from build123d import *

# Parameters (mm, degrees)
SKETCH1_W                                   = 65
SKETCH1_H                                   = 40
BOSS_EXTRUDE1_DEPTH                         = 30
SKETCH3_R                                   = 10
CUT_EXTRUDE2_DEPTH                          = 35
CBORE_FOR_M4_CHEESE_HEAD_SCREW1_D           = 4.5
CBORE_FOR_M4_CHEESE_HEAD_SCREW1_CBORE_D     = 8
CBORE_FOR_M4_CHEESE_HEAD_SCREW1_CBORE_DEPTH = 2.6
SKETCH10_R                                  = 2.25
CUT_EXTRUDE8_DEPTH                          = 4
CUT_EXTRUDE9_DEPTH                          = 15
CUT_EXTRUDE10_DEPTH                         = 83.006097414
FILLET9_R                                   = 8
SKETCH12_R                                  = 2.25
CUT_EXTRUDE11_DEPTH                         = 8
SKETCH12_3_R                                = 2.25
CUT_EXTRUDE12_DEPTH                         = 79.010807554
FILLET10_R                                  = 3


with BuildPart() as part:
    # Sketch1 → Boss-Extrude1 (new body)
    with BuildSketch(Plane(origin=(0, 0, 0), x_dir=(1, 0, 0), z_dir=(0, 1, 0))):
        with Locations((32.5, 20)):
            Rectangle(SKETCH1_W, SKETCH1_H)
    extrude(amount=BOSS_EXTRUDE1_DEPTH)

    # Sketch3 → Cut-Extrude2 (cut)
    with BuildSketch(Plane(origin=(65, 0, 0), x_dir=(0, 0, -1), z_dir=(1, 0, 0))):
        with Locations((20, 15)):
            Circle(SKETCH3_R)
    extrude(amount=-CUT_EXTRUDE2_DEPTH, mode=Mode.SUBTRACT)

    # CBORE for M4 Cheese Head Screw1 (through all)
    with Locations(Plane(origin=(0, 30, 0), x_dir=(1, 0, 0), z_dir=(0, 1, 0))):
        with Locations((53, 20)):
            CounterBoreHole(CBORE_FOR_M4_CHEESE_HEAD_SCREW1_D / 2, CBORE_FOR_M4_CHEESE_HEAD_SCREW1_CBORE_D / 2, CBORE_FOR_M4_CHEESE_HEAD_SCREW1_CBORE_DEPTH)

    # Sketch10 → Cut-Extrude8 (cut)
    with BuildSketch(Plane.XZ):
        Polygon((53, -15.669872981), (49.25, -17.834936491), (49.25, -22.165063509), (53, -24.330127019), (56.75, -22.165063509), (56.75, -17.834936491), align=None)
        with Locations(Location((53, -20, 0), (0, 0, 90))):
            Circle(SKETCH10_R, mode=Mode.SUBTRACT)
    extrude(amount=-CUT_EXTRUDE8_DEPTH, mode=Mode.SUBTRACT)

    # Sketch2 → Cut-Extrude9 (cut)
    with BuildSketch(Plane(origin=(0, 30, 0), x_dir=(1, 0, 0), z_dir=(0, 1, 0))):
        with BuildLine():
            Line((17.014944168, 22.55), (12.985055832, 22.55))
            ThreePointArc((12.985055832, 22.55), (13.583325822, 17.075015509), (18.25, 20))
            ThreePointArc((18.25, 20), (17.924984491, 21.416674178), (17.014944168, 22.55))
        make_face()
    extrude(amount=-CUT_EXTRUDE9_DEPTH, mode=Mode.SUBTRACT)

    # Sketch2<7> → Cut-Extrude10 (cut, through all)
    with BuildSketch(Plane(origin=(0, 30, 0), x_dir=(1, 0, 0), z_dir=(0, 1, 0))):
        with BuildLine():
            Line((65, 40), (0, 40))
            Line((0, 40), (0, 19.999999921))
            ThreePointArc((0, 19.999999921), (4.393398254, 30.60660169), (15, 35))
            add(Edge.make_bspline(
                [(15, 35), (30.758528256, 35), (45.015961289, 29.236867717), (65, 40)],
                knots=[0, 0, 0, 0, 1, 1, 1, 1], degree=3))
        make_face()
        with BuildLine():
            ThreePointArc((15, 5), (4.39339831, 9.393398254), (0, 19.999999921))
            Line((0, 19.999999921), (0, 0))
            Line((0, 0), (65, 0))
            add(Edge.make_bspline(
                [(15, 5), (30.758528256, 5), (45.015961289, 10.763132283), (65, 0)],
                knots=[0, 0, 0, 0, 1, 1, 1, 1], degree=3))
        make_face()
    extrude(amount=-CUT_EXTRUDE10_DEPTH, mode=Mode.SUBTRACT)

    # Fillet9
    # the kernel refuses this fillet: 8 mm, written as the material it takes off along each edge
    with BuildSketch(Plane(origin=(65, 0, -40), x_dir=(0, 0, 1), z_dir=(0, 1, 0))) as fillet9_piece_1:
        with BuildLine():
            CenterArc((12.0050638, -8), FILLET9_R, 90, 106.898701243)
            Line((4.350502414, -10.325444039), (4.197411186, -10.37195292))
            ThreePointArc((4.197411186, -10.37195292), (2.285588644, -5.115947892), (-0.140868031, -0.075869611))
            Line((-0.140868031, -0.075869611), (0, 0.16))
            Line((0, 0.16), (12.0050638, 0.16))
            Line((12.0050638, 0.16), (12.0050638, 0))
        make_face()
    extrude(amount=30, mode=Mode.SUBTRACT)
    with BuildSketch(Plane(origin=(65, 0, 0), x_dir=(0, 0, -1), z_dir=(0, 1, 0))) as fillet9_piece_2:
        with BuildLine():
            CenterArc((12.0050638, 8), FILLET9_R, 163.101298757, 106.898701243)
            Line((4.350502414, 10.325444039), (4.197411186, 10.37195292))
            ThreePointArc((4.197411186, 10.37195292), (2.285588644, 5.115947892), (-0.140868031, 0.075869611))
            Line((-0.140868031, 0.075869611), (0, -0.16))
            Line((0, -0.16), (12.0050638, -0.16))
            Line((12.0050638, -0.16), (12.0050638, 0))
        make_face()
    extrude(amount=30, mode=Mode.SUBTRACT)

    # Sketch12 → Cut-Extrude11 (cut)
    # profile 1 of 2: a face of its own
    with BuildSketch(Plane.XY.offset(-35)):
        Polygon((15, 17.727608008), (18.7, 19.863804004), (18.7, 24.136195996), (15, 26.272391992), (11.3, 24.136195996), (11.3, 19.863804004), align=None)
        with Locations((15, 22)):
            Circle(SKETCH12_R, mode=Mode.SUBTRACT)
    # profile 2 of 2: a face of its own
    with BuildSketch(Plane.XY.offset(-35)):
        with Locations((15, 22)):
            Circle(SKETCH12_R)
    extrude(amount=CUT_EXTRUDE11_DEPTH, mode=Mode.SUBTRACT)

    # Sketch12<3> → Cut-Extrude12 (cut, through all)
    with BuildSketch(Plane.XY.offset(-35)):
        with Locations(Location((15, 22, 0), (0, 0, 153.576683422))):
            Circle(SKETCH12_3_R)
    extrude(amount=CUT_EXTRUDE12_DEPTH, mode=Mode.SUBTRACT)

    # Fillet10
    fillet10_edges = [part.edges().sort_by_distance(p)[0] for p in [
        (0, 30, -20),
        (34.916790613, 30, -33.583596944),
        (34.916790613, 30, -6.416403056),
        (65, 30, -20),
        (61.7642653, 30, -34.421581993),
        (61.7642653, 30, -5.578418007),
    ]]
    fillet(fillet10_edges, radius=FILLET10_R)


solid = part.part
Part model, mm, in its own coordinate system. A direction names the side the tool comes from. Coordinates: 2 decimals unless noted, no trailing zeros. Use a Markdown table: item, result. Add a question column.
Q1. Pin check, flat tips, straight feed: P1, Ø3, axis at x = 58, y = 5, coming from the +Z side; P2, Ø4, axis at x = 54, z = -21, coming from the +Y side; P3, Ø6, axis at y = 17.5, z = -15.5, coming from the +X side; P4, Ø6, axis at x = 53, z = -20, coming from the -Y side. Stop position of each tip, or through.
Q2. Which spindle directions (+Z, -Z, +X, -X, +Y, -Y) get a long thin tool onto all of the face, cutting with end or side? Do faces 1 (the flat face through (16.82, 18.78, -31.06)), 2 (the flat face through (15, 17, -22.55)), 3 (the cylindrical face through (14.96, 24.25, -11.42)), 4 (the flat face through (54.85, 1.97, -23.26)). Say none if no direction does.
Q3. Probe L1, parallel to Y at x = 15, z = -25.45; L2, parallel to Y at x = 55.5, z = -20; L3, parallel to X at y = 16.5, z = -18.5. List the from-to ranges inside material, lowest first.
Q4. Mould opens along X. For faces 5 (the flat face through (51.099, 1.972, -23.232)), 6 (the cylindrical face through (64.1, 29.14, -19.89)), 7 (the flat face through (51, 4, -22)), 8 (the flat face through (32, 30, -20)) say: +X half, -X half, draft (parallel to the pull), parting line (faces both ways), or undercut.
Worked out:
| question | item | result |
|---|---|---|
| 1 | P1 | stops at z = -4.01 |
| 1 | P2 | stops at y = 27.4 |
| 1 | P3 | stops at x = 30 |
| 1 | P4 | stops at y = 4 |
| 2 | face 1 | -Z |
| 2 | face 2 | +Y |
| 2 | face 3 | +Z, -Z |
| 2 | face 4 | -Y |
| 3 | L1 | y = 0 to 19.75, 24.25 to 30 |
| 3 | L2 | y = 4 to 5, 25 to 27.4 |
| 3 | L3 | x = 0.08 to 12.12, 17.88 to 30 |
| 4 | face 5 | undercut |
| 4 | face 6 | +X half |
| 4 | face 7 | undercut |
| 4 | face 8 | draft |
